from build123d import *

# Parameters (mm, degrees)
F1_DEPTH = 2
F2_DEPTH = 6


with BuildPart() as f1:
    # F0 (on Front) → F1 (new body)
    with BuildSketch(Plane.XZ):
        with BuildLine():
            Line((0, 24), (0, 0))
            Line((0, 0), (60, 0))
            Line((60, 0), (60, -10))
            Line((60, -10), (73, -10))
            Line((73, -10), (73, 4.935162))
            ThreePointArc((73, 4.935162), (69.638883, 13.658231), (61.293548, 17.870645))
            Line((61.293548, 17.870645), (0, 24))
        make_face()
        with BuildLine():
            Line((62.5, 2.5), (2.5, 2.5))
            Line((2.5, 2.5), (2.5, 21.237531))
            Line((2.5, 21.237531), (61.044789, 15.383052))
            ThreePointArc((61.044789, 15.383052), (67.785252, 11.980718), (70.5, 4.935162))
            Line((70.5, 4.935162), (70.5, -7.5))
            Line((70.5, -7.5), (62.5, -7.5))
            Line((62.5, -7.5), (62.5, 2.5))
        make_face(mode=Mode.SUBTRACT)
        with BuildLine():
            Line((2.5, 21.237531), (2.5, 2.5))
            Line((2.5, 2.5), (62.5, 2.5))
            Line((62.5, 2.5), (62.5, -7.5))
            Line((62.5, -7.5), (70.5, -7.5))
            Line((70.5, -7.5), (70.5, 4.935162))
            ThreePointArc((70.5, 4.935162), (67.785252, 11.980718), (61.044789, 15.383052))
            Line((61.044789, 15.383052), (2.5, 21.237531))
        make_face()
    extrude(amount=-F1_DEPTH)

    # F0 (on Front) → F2 (join)
    with BuildSketch(Plane.XZ):
        with BuildLine():
            Line((2.5, 21.237531), (2.5, 2.5))
            Line((2.5, 2.5), (62.5, 2.5))
            Line((62.5, 2.5), (62.5, -7.5))
            Line((62.5, -7.5), (70.5, -7.5))
            Line((70.5, -7.5), (70.5, 4.935162))
            ThreePointArc((70.5, 4.935162), (67.785252, 11.980718), (61.044789, 15.383052))
            Line((61.044789, 15.383052), (2.5, 21.237531))
        make_face()
    extrude(amount=F2_DEPTH)


solid = f1.part
For this review, take the finished solid that the model builds, in its own axes (mm). A direction names the side the tool comes from. Give positions to 0.01 mm unless a question says otherwise; leave off trailing zeros. Loops run counter-clockwise (first coordinate to the right, second up) from the corner with the lowest first, then second, coordinate; pieces in that order, holes last.
Item 1: Take a section at A-A, the plane y = 0.75. State the section outline as (x, z) points, and give its area (3 significant figures).
Item 2: Take a section at B-B, the plane z = 11. State the section outline as (x, y) points.
Item 3: For line 1 along X through (y, z) = (-2, -0.5); line 2 along Y through (x, z) = (17.5, 2); line 3 along X through (y, z) = (-5, 4), list the stretches that pass through material, from the lowest coordinate up.
Item 4: Tool access review of faces 1 (the flat face through (66, -3, -7.5)), 2 (the flat face through (32, -3, 2.5)), 3 (the cylindrical face through (67.86, -2.96, 11.9)): name each direction out of +Z, -Z, +X, -X, +Y, -Y from which nothing blocks a thin tool from reaching the whole face with its end or side.
Item 5: Take a section at C-C, the plane x = 43. State the section outline as (y, z) points.
Item 6: Insertion check: pin 1 (2 mm diameter, centred on x = 22, y = 1, fed in from -Z); pin 2 (0.6 mm diameter, centred on y = 1, z = -6.5, fed in from -X); pin 3 (3 mm diameter, centred on x = 18, y = -2.5, fed in from -Z). Each pin has a flat end and moves straight along its axis. Give the tip position at first contact, or say it passes through.
Calculated:
1. outline: (0, 0) - (60, 0) - (60, -10) - (73, -10) - (73, 4.94) arc R13 ccw to (61.29, 17.87) - (0, 24) - close
1. area: 1,590 mm2
2. outline: (0, 0) - (2.5, 0) - (2.5, -6) - (68.57, -6) - (68.57, 0) - (71.5, 0) - (71.5, 2) - (0, 2) - close
3. line 1: x = 62.5 to 70.5
3. line 2: y = 0 to 2
3. line 3: x = 2.5 to 70.5
4. face 1: -Z, +X, -X, -Y
4. face 2: -Z, -X, -Y
4. face 3: +Z, +X, -Y
5. outline: (-6, 2.5) - (0, 2.5) - (0, 0) - (2, 0) - (2, 19.7) - (0, 19.7) - (0, 17.19) - (-6, 17.19) - close
6. pin 1: stops at z = 0
6. pin 2: stops at x = 60
6. pin 3: stops at z = 2.5
